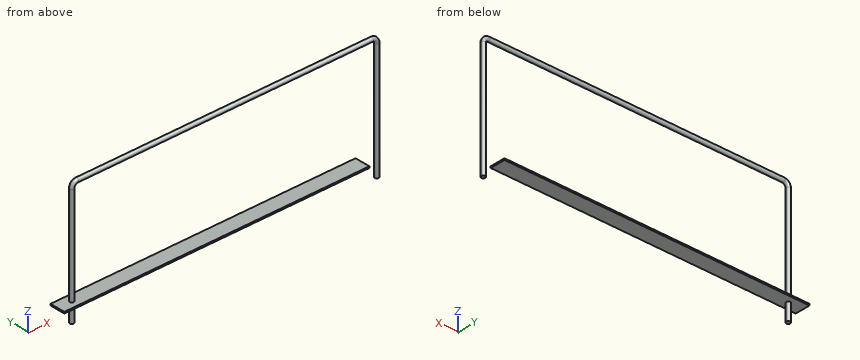
from build123d import *

# Parameters (mm, degrees)
F1_R     = 5.08
F3_W     = 38.1
F3_H     = 3.81
F4_DEPTH = 381


with BuildPart() as f2:
    # F2: sweep along a path in F0
    with BuildLine(Plane.XZ) as f2_path:
        Line((-345.471335, 0), (-345.471335, 292.1))
        ThreePointArc((-345.471335, 292.1), (-341.751591, 301.080256), (-332.771335, 304.8))
        Line((-332.771335, 304.8), (403.828665, 304.8))
        ThreePointArc((403.828665, 304.8), (412.808921, 301.080256), (416.528665, 292.1))
        Line((416.528665, 292.1), (416.528665, 0))
    # F1 (on Top) → F2 (sweep)
    with BuildSketch(Plane.XY):
        with Locations((-345.471335, 0)):
            Circle(F1_R)
    sweep(path=f2_path.line)

    # F3 (on Right) → F4 (join, symmetric)
    with BuildSketch(Plane.YZ):
        with Locations((0.267047, 44.76991)):
            Rectangle(F3_W, F3_H)
    extrude(amount=F4_DEPTH, both=True)


solid = f2.part
Design review of the part built by this model. Coordinates are the model's own, in mm. Round coordinates to 2 decimals unless told otherwise and drop trailing zeros. Loops run counter-clockwise (first coordinate to the right, second up) from the corner with the lowest first, then second, coordinate; pieces in that order, holes last. Notation, with made-up numbers: (33, 34) - (78, 34) arc R10 ccw to (78, 48) - close; hole circle Ø7 at (-24.75, -0.5). An arc over 180 degrees is marked (long way). One line per item, written item: value. Start each with the question number.
1) To check wall thickness, follow L1, parallel to Z at x = -198.5, y = 1; L2, parallel to X at y = -1, z = 222; L3, parallel to X at y = 0.5, z = 134.5. State the ranges of each line that lie inside material, in increasing order. Write a range as from..to.
2) Insertion check: pin 1 Ø11.5 at (x, y) = (-179, 1) entering from -Z; pin 2 Ø3 at (y, z) = (-7, 44) entering from +X; pin 3 Ø12 at (x, y) = (17, -8) entering from +Z. Each pin has a flat end and moves straight along its axis. Give the tip position at first contact, or say it passes through.
3) Consider section A-A on y = -11.5. Give the boundary of the cut face in (x, z).
Reported:
1. L1: z = 42.86..46.67, 299.82..309.78
1. L2: x = -350.45..-340.49, 411.55..421.51
1. L3: x = -350.53..-340.42, 411.47..421.58
2. pin 1: stops at z = 42.86
2. pin 2: stops at x = 381
2. pin 3: stops at z = 309.47
3. outline: (-381, 42.86) - (381, 42.86) - (381, 46.67) - (-381, 46.67) - close
